```python
from build123d import *

# Parameters (mm, degrees)
SKETCH1_W               = 181.7773
SKETCH1_H               = 180
BOSS_EXTRUDE1_DEPTH     = 3
SKETCH2_W               = 16.797936363
SKETCH2_H               = 3
SKETCH2_W_2             = 16.797936364
SKETCH2_W_3             = 3
SKETCH2_H_2             = 20
BOSS_EXTRUDE2_DEPTH     = 3
SKETCH3_W               = 164.7773
SKETCH3_H               = 80
CUT_EXTRUDE1_DEPTH      = 1
CUT_EXTRUDE1_DEPTH_BACK = 4
FILLET1_R               = 15
CUT_EXTRUDE2_DEPTH      = 10


with BuildPart() as part:
    # Sketch1 → Boss-Extrude1 (new body)
    with BuildSketch(Plane(origin=(0, 0, 0), x_dir=(0, 0, -1), z_dir=(1, 0, 0))):
        Rectangle(SKETCH1_W, SKETCH1_H)
    extrude(amount=BOSS_EXTRUDE1_DEPTH)

    # Sketch2 → Boss-Extrude2 (add)
    with BuildSketch(Plane(origin=(3, 0, 0), x_dir=(0, 0, -1), z_dir=(1, 0, 0))):
        with Locations((-65.691745455, -91.5)):
            Rectangle(SKETCH2_W, SKETCH2_H)
        with Locations((-32.095872727, -91.5)):
            Rectangle(SKETCH2_W_2, SKETCH2_H)
        with Locations((1.5, -91.5)):
            Rectangle(SKETCH2_W_2, SKETCH2_H)
        with Locations((92.38865, -60)):
            Rectangle(SKETCH2_W_3, SKETCH2_H_2)
        with Locations((92.38865, -20)):
            Rectangle(SKETCH2_W_3, SKETCH2_H_2)
        with Locations((92.38865, 20)):
            Rectangle(SKETCH2_W_3, SKETCH2_H_2)
        with Locations((92.38865, 60)):
            Rectangle(SKETCH2_W_3, SKETCH2_H_2)
        with Locations((-92.38865, -60)):
            Rectangle(SKETCH2_W_3, SKETCH2_H_2)
        with Locations((-92.38865, -20)):
            Rectangle(SKETCH2_W_3, SKETCH2_H_2)
        with Locations((-92.38865, 20)):
            Rectangle(SKETCH2_W_3, SKETCH2_H_2)
        with Locations((-92.38865, 60)):
            Rectangle(SKETCH2_W_3, SKETCH2_H_2)
        with Locations((35.095872727, -91.5)):
            Rectangle(SKETCH2_W_2, SKETCH2_H)
        with Locations((68.691745455, -91.5)):
            Rectangle(SKETCH2_W, SKETCH2_H)
    extrude(amount=-BOSS_EXTRUDE2_DEPTH)

    # Sketch3 → Cut-Extrude1 (cut, two sides)
    with BuildSketch(Plane(origin=(3, 0, 0), x_dir=(0, 0, -1), z_dir=(1, 0, 0))) as cut_extrude1_sk:
        with Locations((11.5, 50)):
            Rectangle(SKETCH3_W, SKETCH3_H)
    extrude(amount=CUT_EXTRUDE1_DEPTH, mode=Mode.SUBTRACT)
    extrude(cut_extrude1_sk.sketch, amount=-CUT_EXTRUDE1_DEPTH_BACK, mode=Mode.SUBTRACT)

    # Fillet1
    fillet1_edges = [part.edges().sort_by_distance(p)[0] for p in [
        (1.5, 10, 70.88865),
        (1.5, 90, 70.88865),
    ]]
    fillet(fillet1_edges, radius=FILLET1_R)

    # Sketch4 → Cut-Extrude2 (cut)
    with BuildSketch(Plane.ZY):
        Polygon((-67.83865663, -65.5), (-81.88865, -65.5), (-81.88865, -78), (-60.621778265, -78), align=None)
        Polygon((-49.074772881, -43), (-59.178402592, -60.5), (-49.074772881, -78), (-28.867513459, -78), (-18.763883749, -60.5), (-28.867513459, -43), align=None)
        Polygon((-10.103629711, -65.5), (-17.320508076, -78), (17.320508076, -78), (10.103629711, -65.5), align=None)
        Polygon((28.867513459, -43), (18.763883749, -60.5), (28.867513459, -78), (49.074772881, -78), (59.178402592, -60.5), (49.074772881, -43), align=None)
        Polygon((81.88865, -78), (81.88865, -65.5), (67.83865663, -65.5), (60.621778265, -78), align=None)
        Polygon((81.88865, -55.5), (81.88865, -20.5), (67.83865663, -20.5), (57.735026919, -38), (67.83865663, -55.5), align=None)
        Polygon((51.384173958, -2), (26.558112383, -2), (18.763883749, -15.5), (28.867513459, -33), (49.074772881, -33), (59.178402592, -15.5), align=None)
        Polygon((81.88865, -10.5), (81.88865, -2), (62.931179342, -2), (67.83865663, -10.5), align=None)
        Polygon((20.207259422, -38), (10.103629711, -20.5), (-10.103629711, -20.5), (-20.207259422, -38), (-10.103629711, -55.5), (10.103629711, -55.5), align=None)
        Polygon((15.011106999, -2), (-15.011106999, -2), (-10.103629711, -10.5), (10.103629711, -10.5), align=None)
        Polygon((-26.558112383, -2), (-51.384173958, -2), (-59.178402592, -15.5), (-49.074772881, -33), (-28.867513459, -33), (-18.763883749, -15.5), align=None)
        Polygon((-67.83865663, -20.5), (-81.88865, -20.5), (-81.88865, -55.5), (-67.83865663, -55.5), (-57.735026919, -38), align=None)
        Polygon((-62.931179342, -2), (-81.88865, -2), (-81.88865, -10.5), (-67.83865663, -10.5), align=None)
    extrude(amount=-CUT_EXTRUDE2_DEPTH, mode=Mode.SUBTRACT)


solid = part.part
```
Can you work these out from the model? Positions are in its coordinate system, mm. A direction names the side the tool comes from. Round coordinates to 2 decimals unless told otherwise and drop trailing zeros. Loops run counter-clockwise (first coordinate to the right, second up) from the corner with the lowest first, then second, coordinate; pieces in that order, holes last.
Item 1: Please list where these lines run through material, in increasing order: L1, parallel to Y at x = 0.2, z = 33; L2, parallel to Y at x = 1.9, z = -69; L3, parallel to Y at x = 2.25, z = 7.5.
Item 2: Suppose I cut it at C-C, the plane x = 2.4. State how many separate pieces and enclosed holes the cut face has, then the cut area to 4 significant figures.
Item 3: Suppose I cut it at B-B, the plane y = -6. Write out the boundary of the cut face in (x, z).
Item 4: Will this pin go through, and if not, where does the flat tip stop? pin 1 Ø0.9 at (x, z) = (1, 41.5) entering from -Y.
Item 5: Which directions (+Z, -Z, +X, -X, +Y, -Y) give clear straight access to the entire face, cutting with the end or side of a thin tool? Please do faces 5 (the flat face through (1.479, -24.372, 54.056)), 6 (the flat face through (3, -41, 22)).
Item 6: If we mould it in two halves opening along Y, with no side actions, what happens to faces 1 (the flat face through (1.479, -69.128, -54.197)), 2 (the flat face through (1.479, -46.872, -62.858)), 3 (the flat face through (0, -41, 22)), 4 (the cylindrical face through (1.479, 85.723, 75.399))? For each: +Y half, -Y half, draft (parallel to the pull), parting line (faces both ways), or undercut.
Item 7: Suppose I cut it at A-A, the plane z = 4.5. Write out the boundary of the cut face in (x, y), then the cut area to 3 significant figures.
Reported:
1. L1: y = -93 to -78, -43 to -33, -2 to 10
1. L2: y = -93 to -78, -65.5 to -55.5, -20.5 to -10.5, -2 to 10
1. L3: y = -90 to -78, -65.5 to -55.5, -20.5 to -10.5, -2 to 10
2. separate pieces: 1
2. enclosed holes: 13
2. area: 12,650 mm2
3. outline: (0, -90.89) - (3, -90.89) - (3, -81.89) - (0, -81.89) - close; (0, -65.24) - (3, -65.24) - (3, -53.69) - (0, -53.69) - close; (0, -24.25) - (3, -24.25) - (3, -12.7) - (0, -12.7) - close; (0, 12.7) - (3, 12.7) - (3, 24.25) - (0, 24.25) - close; (0, 53.69) - (3, 53.69) - (3, 65.24) - (0, 65.24) - close; (0, 81.89) - (3, 81.89) - (3, 90.89) - (0, 90.89) - close
4. pin 1: stops at y = -90
5. face 5: +X, -X
5. face 6: +Z, -Z, +X, +Y, -Y
6. face 1: undercut
6. face 2: undercut
6. face 3: draft
6. face 4: +Y half
7. outline: (0, -93) - (3, -93) - (3, -78) - (0, -78) - close; (0, -65.5) - (3, -65.5) - (3, -55.5) - (0, -55.5) - close; (0, -20.5) - (3, -20.5) - (3, -10.5) - (0, -10.5) - close; (0, -2) - (3, -2) - (3, 10) - (0, 10) - close
7. area: 141 mm2
